Geometry check sheet. Reference: the model listing, model coordinates, mm. A direction names the side the tool comes from. Round coordinates to 2 decimals unless told otherwise and drop trailing zeros. Loops run counter-clockwise (first coordinate to the right, second up) from the corner with the lowest first, then second, coordinate; pieces in that order, holes last. Notation, with made-up numbers: (39.25, 17.25) - (57.25, 17.25) arc R24 cw to (57.25, 46.25) - close; hole circle Ø4 at (-33.75, 18.5). An arc over 180 degrees is marked (long way). Write item = value, one per line.
```python
from build123d import *

# Parameters (mm, degrees)
F0_R     = 47.4599930616
F0_R_2   = 5.4133355618
F0_R_3   = 5.4163453987
F0_R_4   = 4.4383518645
F0_R_5   = 28.344153959
F0_R_6   = 5.55874857
F1_DEPTH = 25.4
F2_R     = 28.4576632657
F3_DEPTH = 101.6
F4_SIZE  = 25.4


# Not quite as in the source:
# - a fillet or chamfer that OpenCascade refuses, or shapes differently, is made with other operations: its cross-section is extruded or revolved along the edge and cut away or added


with BuildPart() as f1:
    # F0 (on Front) → F1 (new body)
    with BuildSketch(Plane.XZ):
        Circle(F0_R)
        with Locations((-34.2844575644, -17.503157258)):
            Circle(F0_R_2, mode=Mode.SUBTRACT)
        with Locations((28.3297896385, -24.3600457907)):
            Circle(F0_R_3, mode=Mode.SUBTRACT)
        with Locations((-18.9466699958, 31.7582041025)):
            Circle(F0_R_4, mode=Mode.SUBTRACT)
        Circle(F0_R_5, mode=Mode.SUBTRACT)
        with Locations((23.2773423195, 29.0515273809)):
            Circle(F0_R_6, mode=Mode.SUBTRACT)
    extrude(amount=F1_DEPTH)

    # F2 (on Front) → F3 (join)
    with BuildSketch(Plane.XZ):
        Circle(F2_R)
    extrude(amount=F3_DEPTH)

    # F4
    f4_edges = [f1.edges().sort_by_distance(p)[0] for p in [
        (-28.457663, -101.6, 0),
    ]]
    chamfer(f4_edges, length=F4_SIZE)

    # F5: fillet of radius 5.08 on 1 edges, made by hand

    # F5_s1 → F5_t2 (revolve, cut)
    with BuildSketch(Plane.XY):
        with BuildLine():
            ThreePointArc((42.3799930616, -25.4), (45.9720955101, -23.9121024484), (47.4599930616, -20.32))
            Line((47.4599930616, -20.32), (47.4599930616, -25.4))
            Line((47.4599930616, -25.4), (42.3799930616, -25.4))
        make_face()
    revolve(axis=Axis((0, -25.4, 0), (0, -1, 0)), mode=Mode.SUBTRACT)


solid = f1.part
```
(1) Scan lines: L1, parallel to X at y = -5.5, z = 28.5; L2, parallel to Y at x = 35, z = 17.5; L3, parallel to Z at x = 38, y = -10.5. Record each from-to range of solid material in increasing order. Write a range as [from, to].
Answers follow:
L1 = [-37.95, -21.96], [-15.93, 17.75], [28.81, 37.95]
L2 = [-25.4, 0]
L3 = [-28.43, 28.43]
(2) Section check A-A (x = 0). Enter the section's corners in (y, z), then the cut area to 3 significant figures.
Answers follow:
outline = (-101.6, -3.06) - (-76.2, -28.46) - (-25.4, -28.46) - (-25.4, -42.38) arc R5.08 ccw to (-20.32, -47.46) - (0, -47.46) - (0, 47.46) - (-20.32, 47.46) arc R5.08 ccw to (-25.4, 42.38) - (-25.4, 28.46) - (-76.2, 28.46) - (-101.6, 3.06) - close
area = 6,090 mm²
(3) Set-up check for faces 1 (the flat face through (-10, -25.4, -28)), 2 (the cylindrical face through (28.41, -12.52, 26.92)): record each of +Z, -Z, +X, -X, +Y, -Y from which the full face is reachable in a straight line by a thin tool's end or side.
Answers follow:
face_1 = -Y
face_2 = +Y, -Y
(4) Section check C-C (y = -22). Enter the section's corners in (x, z).
Answers follow:
outline = circle Ø94.35 at (0, 0); hole circle Ø10.83 at (-34.28, -17.5); hole circle Ø8.88 at (-18.95, 31.76); hole circle Ø11.12 at (23.28, 29.05); hole circle Ø10.83 at (28.33, -24.36)
(5) Gauge pin test, flat ends, axial feed: pin 1 (1 mm diameter, centred on y = -55.5, z = -15, fed in from +X); pin 2 (5 mm diameter, centred on x = 4.5, z = -10, fed in from -Y); pin 3 (3 mm diameter, centred on x = -16, z = -28.5, fed in from -Y). Record the tip position at first contact, or that the pin passes through.
Answers follow:
pin_1 = 24.49
pin_2 = -96.19
pin_3 = -25.4
(6) Mould release check, pull along X, two halves, no side actions. Record for faces 3 (the cylindrical face through (-29.12, -12.52, -15.88)), 4 (the flat face through (0, -101.6, 0)), 5 (the cylindrical face through (31.24, -12.52, -19.79)), 6 (the cylindrical face through (-6.178, -10.018, 47.056)): pulls with the +X half, pulls with the -X half, needs draft (parallel to the pull), parting line crosses it, or undercut.
Answers follow:
face_3 = undercut
face_4 = needs draft
face_5 = undercut
face_6 = parting line crosses it
(7) Section check B-B (z = 0). Enter the section's corners in (x, y), then the cut area to 3 significant figures.
Answers follow:
outline = (-47.46, -20.32) arc R5.08 ccw to (-42.38, -25.4) - (-28.46, -25.4) - (-28.46, -76.2) - (-3.06, -101.6) - (3.06, -101.6) - (28.46, -76.2) - (28.46, -25.4) - (42.38, -25.4) arc R5.08 ccw to (47.46, -20.32) - (47.46, 0) - (-47.46, 0) - close
area = 6,090 mm²
(8) Section check D-D (y = -51.5). Enter the section's corners in (x, z).
Answers follow:
outline = circle Ø56.92 at (0, 0)
